```python
from build123d import *

# Parameters (mm, degrees)
SKETCH_6_R          = 14.593002621
CUT_EXTRUDE_2_DEPTH = 12


with BuildPart() as part:
    # 草图4 → 旋转2 (revolve)
    with BuildSketch(Plane.XY, mode=Mode.PRIVATE) as revolve_2_sk:
        with BuildLine():
            Line((0, 85), (0, 0))
            Line((0, 0), (25, 0))
            Line((25, 0), (25, 4.109275191))
            ThreePointArc((25, 4.109275191), (24.827000127, 4.92295236), (24.337929463, 5.595863483))
            Line((24.337929463, 5.595863483), (15.570457453, 13.486588292))
            ThreePointArc((15.570457453, 13.486588292), (14.949055524, 13.867240823), (14.23252799, 14))
            Line((14.23252799, 14), (6, 14))
            Line((6, 14), (6, 24.2))
            Line((6, 24.2), (10.235, 24.2))
            Line((10.235, 24.2), (10.235, 35))
            Line((10.235, 35), (6, 35))
            Line((6, 35), (5, 35.75155816))
            Line((5, 35.75155816), (6, 36.503116319))
            Line((6, 36.503116319), (5, 37.254674479))
            Line((5, 37.254674479), (6, 38.006232638))
            Line((6, 38.006232638), (5, 38.757790798))
            Line((5, 38.757790798), (6, 39.509348958))
            Line((6, 39.509348958), (5, 40.260907117))
            Line((5, 40.260907117), (6, 41.012465277))
            Line((6, 41.012465277), (5, 41.764023436))
            Line((5, 41.764023436), (6, 42.515581596))
            Line((6, 42.515581596), (5, 43.267139755))
            Line((5, 43.267139755), (6, 44.018697915))
            Line((6, 44.018697915), (5, 44.770256075))
            Line((5, 44.770256075), (6, 45.521814234))
            Line((6, 45.521814234), (5, 46.273372394))
            Line((5, 46.273372394), (6, 47.024930553))
            Line((6, 47.024930553), (5, 47.776488713))
            Line((5, 47.776488713), (6, 48.528046873))
            Line((6, 48.528046873), (5, 49.279605032))
            Line((5, 49.279605032), (6, 50.031163192))
            Line((6, 50.031163192), (5, 50.782721351))
            Line((5, 50.782721351), (6, 51.534279511))
            Line((6, 51.534279511), (5, 52.285837671))
            Line((5, 52.285837671), (6, 53.03739583))
            Line((6, 53.03739583), (5, 53.78895399))
            Line((5, 53.78895399), (6, 54.540512149))
            Line((6, 54.540512149), (5, 55.292070309))
            Line((5, 55.292070309), (6, 56.043628468))
            Line((6, 56.043628468), (5, 56.795186628))
            Line((5, 56.795186628), (6, 57.546744788))
            Line((6, 57.546744788), (5, 58.298302947))
            Line((5, 58.298302947), (6, 59.049861107))
            Line((6, 59.049861107), (5, 59.801419266))
            Line((5, 59.801419266), (6, 60.552977426))
            Line((6, 60.552977426), (5, 61.304535586))
            Line((5, 61.304535586), (6, 62.056093745))
            Line((6, 62.056093745), (5, 62.807651905))
            Line((5, 62.807651905), (6, 63.559210064))
            Line((6, 63.559210064), (5, 64.310768224))
            Line((5, 64.310768224), (6, 65.062326384))
            Line((6, 65.062326384), (5, 65.813884543))
            Line((5, 65.813884543), (6, 66.565442703))
            Line((6, 66.565442703), (5, 67.317000862))
            Line((5, 67.317000862), (6, 68.068559022))
            Line((6, 68.068559022), (5, 68.820117181))
            Line((5, 68.820117181), (6, 69.571675341))
            Line((6, 69.571675341), (5, 70.323233501))
            Line((5, 70.323233501), (6, 71.07479166))
            Line((6, 71.07479166), (5, 71.82634982))
            Line((5, 71.82634982), (6, 72.577907979))
            Line((6, 72.577907979), (5, 73.329466139))
            Line((5, 73.329466139), (6, 74.081024299))
            Line((6, 74.081024299), (5, 74.832582458))
            Line((5, 74.832582458), (6, 75.584140618))
            Line((6, 75.584140618), (5, 76.335698777))
            Line((5, 76.335698777), (6, 77.087256937))
            Line((6, 77.087256937), (5, 77.838815097))
            Line((5, 77.838815097), (6, 78.590373256))
            Line((6, 78.590373256), (5, 79.341931416))
            Line((5, 79.341931416), (6, 80.093489575))
            Line((6, 80.093489575), (5, 80.845047735))
            Line((5, 80.845047735), (6, 81.596605894))
            Line((6, 81.596605894), (5, 82.348164054))
            Line((5, 82.348164054), (6, 83.099722214))
            Line((6, 83.099722214), (5, 83.851280373))
            Line((5, 83.851280373), (5.655827282, 84.344172718))
            Line((5.655827282, 84.344172718), (5, 85))
            Line((5, 85), (0, 85))
        make_face()
    revolve(revolve_2_sk.sketch.rotate(Axis((0, 84.344172718, 0), (0, 1, 0)), 270), axis=Axis((0, 84.344172718, 0), (0, 1, 0)))

    # 草图6 → 切除-拉伸2 (cut)
    with BuildSketch(Plane(origin=(0, 35, 0), x_dir=(1, 0, 0), z_dir=(0, 1, 0))):
        Circle(SKETCH_6_R)
        Polygon((10.235, 0), (5.1175, 8.863770008), (-5.1175, 8.863770008), (-10.235, 0), (-5.1175, -8.863770008), (5.1175, -8.863770008), align=None, mode=Mode.SUBTRACT)
    extrude(amount=-CUT_EXTRUDE_2_DEPTH, mode=Mode.SUBTRACT)


solid = part.part
```
Source: CAD feature listing. Evaluate the final solid. Frame: model axes, mm. A direction names the side the tool comes from. Give positions to 0.01 mm unless a question says otherwise; leave off trailing zeros. Order: outer loops, then holes, each group sorted by start corner. A loop starts at its lowest first (then second) coordinate and runs counter-clockwise, first axis right, second up.
(1) Pull-direction query (Y, two-part tool) for faces 1 (the face through (1.802, 19.171, 5.723)), 2 (the face through (0, 30, 8.864)), 3 (the face through (-14.191, 13.103, 7.381)); classes: +Y half, -Y half, draft (parallel to the pull), parting line (faces both ways), or undercut.
(2) Section query A-A (y = 25.5). Return the cut outline in (x, z) (1 decimal), plus the area to 3 significant figures.
(3) Access query for faces 4 (the face through (0, 85, 0)), 5 (the face through (-2, 35, -6)). Directions: +Z, -Z, +X, -X, +Y, -Y. A direction counts if a zero-diameter tool reaches every point of the face in a straight line with its end or side. Return the directions, or none.
(4) Section query B-B (y = 16.5). Return the cut outline in (x, z).
(5) Contact query for flat-ended pins moving along their axis: P1, Ø8, axis at x = -2, y = 31, coming from the +Z side; P2, Ø11.5, axis at x = -1, y = 28, coming from the -Z side; P3, Ø6, axis at y = 40.5, z = -3, coming from the +X side. Output: stop coordinate, or through.
(6) Material intervals for line 1 along Y through (x, z) = (-4.5, -10.5); line 2 along Y through (x, z) = (-20, -7); line 3 along X through (y, z) = (5, 22.5), sorted ascending.
Outcome:
1. face 1: undercut
1. face 2: draft
1. face 3: +Y half
2. outline: (-10.2, 0) - (-5.1, -8.9) - (5.1, -8.9) - (10.2, 0) - (5.1, 8.9) - (-5.1, 8.9) - close
2. area: 272 mm2
3. face 4: +Z, -Z, +X, -X, +Y
3. face 5: +Y
4. outline: circle Ø12 at (0, 0)
5. P1: stops at z = 8.86
5. P2: stops at z = -8.86
5. P3: stops at x = 6
6. line 1: y = 0 to 14
6. line 2: y = 0 to 8.43
6. line 3: x = -10.41 to 10.41
